Can you work these out from the model? Positions are in its coordinate system, mm. Round coordinates to 2 decimals unless told otherwise and drop trailing zeros. Loops run counter-clockwise (first coordinate to the right, second up) from the corner with the lowest first, then second, coordinate; pieces in that order, holes last. Notation, with made-up numbers: (-9, 79.5) -> (31, 79.5) arc R23 ccw to (31, 106.5) -> close; hole circle Ø4 at (1, 34). An arc over 180 degrees is marked (long way). Write item = value, one per line.
from build123d import *

# Parameters (mm, degrees)
SKETCH1_R           = 2
BOSS_EXTRUDE1_DEPTH = 2


with BuildPart() as part:
    # Sketch1 → Boss-Extrude1 (new body)
    with BuildSketch(Plane.XY):
        with BuildLine():
            Line((-1.2887257, 9.27170727), (-31.0207003, 8.828891045))
            ThreePointArc((-31.0207003, 8.828891045), (-37.4360697, 0.196784564), (-27.320647525, -3.456770014))
            ThreePointArc((-27.320647525, -3.456770014), (-17.039618289, -1.022120458), (-7.632023625, -5.830887792))
            ThreePointArc((-7.632023625, -5.830887792), (7.224276423, -3.332674299), (-1.0207003, 9.275699134))
            Line((-1.0207003, 9.275699134), (-1.2887257, 9.27170727))
        make_face()
        with BuildLine():
            ThreePointArc((-28.701264232, -1.372568126), (-35.044639656, 0.925598871), (-31.004247939, 6.328858821))
            Line((-31.004247939, 6.328858821), (-1.231370803, 6.772284233))
            ThreePointArc((-1.231370803, 6.772284233), (-7.016861205, 2.784893108), (-5.795544924, -4.134613646))
            ThreePointArc((-5.795544924, -4.134613646), (-16.740328258, 1.459899985), (-28.701264232, -1.372568126))
        make_face(mode=Mode.SUBTRACT)
        with Locations((-1.0207003, 0.275699134)):
            Circle(SKETCH1_R, mode=Mode.SUBTRACT)
        with BuildLine():
            ThreePointArc((1.370109873, 4.088050996), (2.354151579, 7.175485919), (4.9792997, 5.275699134))
            ThreePointArc((4.9792997, 5.275699134), (4.07225701, 3.60075307), (2.173855381, 3.44505459))
            ThreePointArc((2.173855381, 3.44505459), (1.729909605, 3.713961516), (1.370109873, 4.088050996))
        make_face(mode=Mode.SUBTRACT)
    extrude(amount=BOSS_EXTRUDE1_DEPTH)


solid = part.part
1. I need wall thicknesses on line 1 (X direction, y = 4.25, z = 1.5); line 2 (X direction, y = 4, z = 0.7); line 3 (X direction, y = -0.75, z = 1.2). Which ranges of each line are inside material? Lowest first, please. Write a range as [from, to].
Entries:
line_1 = [-37.38, -34.65], [-6.16, 1.26], [4.7, 7.05]
line_2 = [-37.45, -34.78], [-6.35, 1.44], [4.52, 7.17]
line_3 = [-37.07, -34.08], [-27.69, -10.05], [-7.44, -2.74], [0.7, 7.92]
2. Suppose I cut it at C-C, the plane x = -4.5. List the corners of the cut face in (y, z) for me.
Entries:
outline = (-8.02, 0) -> (5.77, 0) -> (5.77, 2) -> (-8.02, 2) -> close; (6.72, 0) -> (9.22, 0) -> (9.22, 2) -> (6.72, 2) -> close
3. I'm going to push flat-ended pins straight in: pin 1 (2.5 mm diameter, centred on x = -1.02, y = 0.28, fed in from -Z); pin 2 (1.5 mm diameter, centred on x = -21, y = 6.5, fed in from -Z). Where does each tip first touch, or does it pass through?
Entries:
pin_1 = through
pin_2 = 0
4. Suppose I cut it at D-D, the plane y = 8. List the corners of the cut face in (x, z) for me, and give its area (3 significant figures).
Entries:
outline = (-34.25, 0) -> (3.6, 0) -> (3.6, 2) -> (-34.25, 2) -> close
area = 75.7 mm²
5. Suppose I cut it at A-A, the plane x = -25. List the corners of the cut face in (y, z) for me, and give its area (3 significant figures).
Entries:
outline = (-2.19, 0) -> (0.5, 0) -> (0.5, 2) -> (-2.19, 2) -> close; (6.42, 0) -> (8.92, 0) -> (8.92, 2) -> (6.42, 2) -> close
area = 10.4 mm²
6. We'd pull the mould along X, two halves only. Please class faces 1 (the cylindrical face through (7.1, -3.6, 1)), 2 (the cylindrical face through (-35.01, 0.82, 0.99)), 3 (the flat face through (-10, -2, 0)): released by +X, released by -X, zero draft, split by the parting line, or undercut.
Entries:
face_1 = split by the parting line
face_2 = undercut
face_3 = zero draft
7. Suppose I cut it at B-B, the plane z = 0.9. List the corners of the cut face in (x, y) for me, and give its area (3 significant figures).
Entries:
outline = (-31.02, 8.83) arc R6.7 ccw (long way) to (-27.32, -3.46) arc R15.3 cw to (-7.63, -5.83) arc R9 ccw (long way) to (-1.02, 9.28) -> close; hole (-31, 6.33) arc R4.2 ccw (long way) to (-28.7, -1.37) arc R17.8 cw to (-5.8, -4.13) arc R6.5 cw to (-1.23, 6.77) -> close; hole circle Ø4 at (-1.02, 0.28); hole circle Ø4 at (2.98, 5.28)
area = 369 mm²
